Geometry: see drawing. Coordinates: mm, zero at the bounding-box minimum. A direction names the side the tool comes from. Coordinates: 2 decimals unless noted, no trailing zeros. Write each loop counter-clockwise with the first axis right and the second up, starting at its lowest first coordinate (ties: lowest second). Pieces come first, ordered by that corner, then holes. Notation, with made-up numbers: (-15, 7) -> (36, 7) arc R23 ccw to (36, 33) -> close; hole circle Ø1 at (48.5, 34). An arc over 180 degrees is marked (long way). Use one line per item in the form item = value. Start each with the question number.
(1) Ray query, line 1 along Z through (x, y) = (165, 79.5); line 2 along Y through (x, z) = (143, 138); line 3 along Y through (x, z) = (135.5, 260). Return the intervals inside material, ascending.
(2) Cut plane C-C on x = 150. Return the cut outline in (y, z) (1 decimal).
(3) Cut plane A-A on y = 200.5. Return the cut outline in (x, z).
(4) Set-up query: the marked faces 5, 6 and 7. Return all of +Z, -Z, +X, -X, +Y, -Y with unobstructed straight access to the full face (end or side cutting, diameter ignored); none if empty.
(5) Pull-direction query (Z, two-part tool) for the marked faces 1, 2, 3 and 4; classes: released by +Z, released by -Z, zero draft, split by the parting line, or undercut.
(6) Cut plane B-B on z = 150. Return the cut outline in (x, y) (1 decimal).
(7) First-contact query: pin 1 (3 mm diameter, centred on y = 31.5, z = 60.5, fed in from +X); pin 2 (4 mm diameter, centred on x = 203, z = 113, fed in from +Y); pin 3 (5 mm diameter, centred on y = 138.5, z = 250, fed in from +X). Flat tips, straight axial feed; report the tip coordinate or a pass-through.
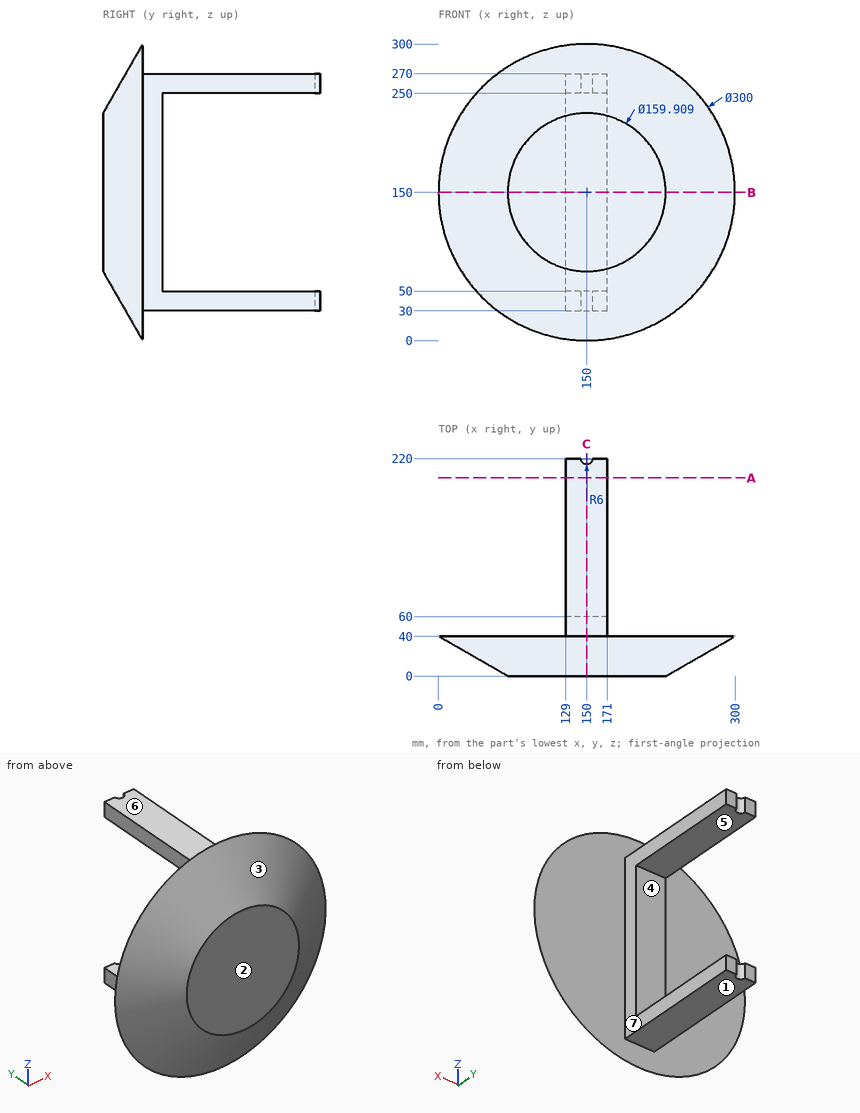
Values:
q1.line_1 = 30 to 50, 250 to 270
q1.line_2 = 0 to 60
q1.line_3 = 17.7 to 220
q2.outline = (0, 70) -> (40, 0) -> (40, 30) -> (214, 30) -> (214, 50) -> (60, 50) -> (60, 250) -> (214, 250) -> (214, 270) -> (40, 270) -> (40, 300) -> (0, 230) -> close
q3.outline = (129, 30) -> (171, 30) -> (171, 50) -> (129, 50) -> close; (129, 250) -> (171, 250) -> (171, 270) -> (129, 270) -> close
q4.face_5 = +X, -X, +Y
q4.face_6 = +Z, +X, -X, +Y
q4.face_7 = +Z, -Z, +X, +Y
q5.face_1 = released by -Z
q5.face_2 = zero draft
q5.face_3 = split by the parting line
q5.face_4 = undercut
q6.outline = (0, 40) -> (70, 0) -> (230, 0) -> (300, 40) -> (171, 40) -> (171, 60) -> (129, 60) -> (129, 40) -> close
q7.pin_1 = 254.93
q7.pin_2 = 40
q7.pin_3 = 171
